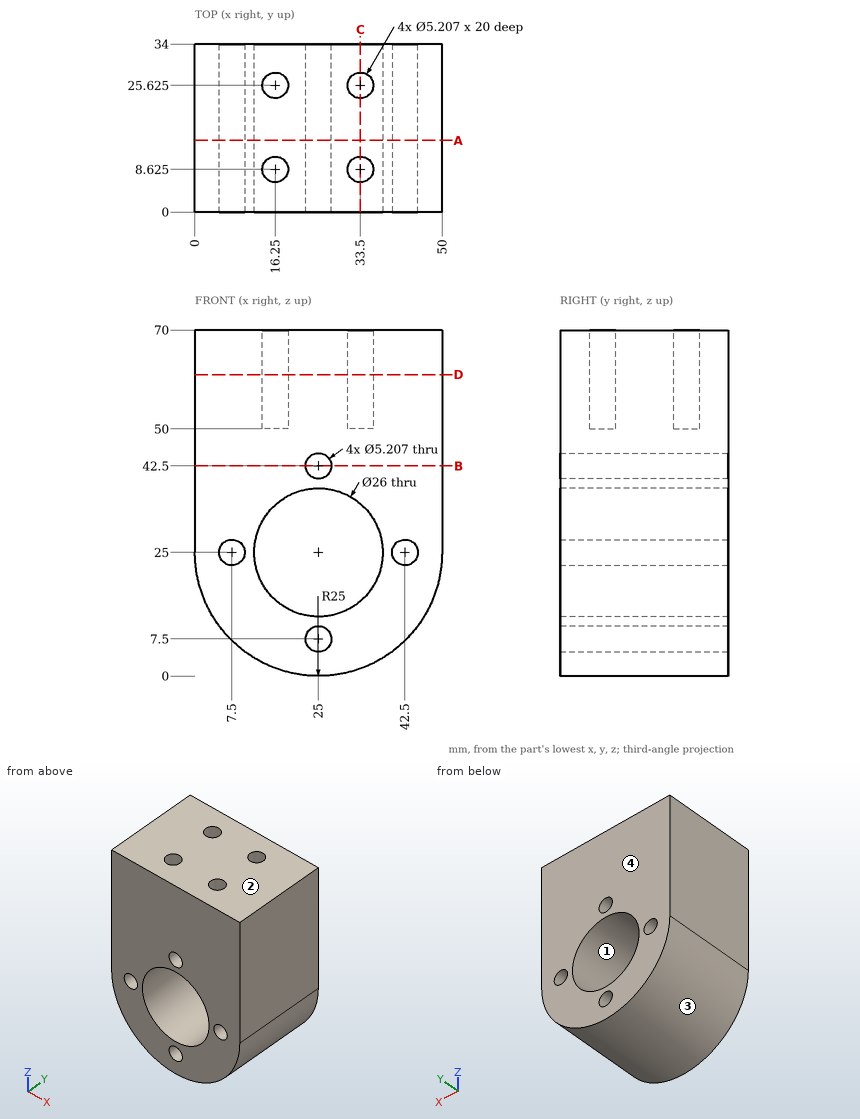
The figure shows three views and two pictorial views of one solid part (mm, origin at its lowest corner). Answer the questions. Round coordinates to 2 decimals unless told otherwise and drop trailing zeros. Loops run counter-clockwise (first coordinate to the right, second up) from the corner with the lowest first, then second, coordinate; pieces in that order, holes last. Notation, with made-up numbers: M 46.5,10.5 L 71.5,10.5 A14 ccw 71.5,35.5 Z; hole C -0.5,-26 d1. An arc over 180 degrees is marked long. Use CSV: the item, a comma, the result in double quotes.
Q1. Each of these flat-tipped pins is pushed along its axis until it touches: pin 1 (12 mm diameter, centred on x = 30.5, z = 15, fed in from +Y); pin 2 (4.5 mm diameter, centred on x = 33.5, y = 8.625, fed in from +Z); pin 3 (4 mm diameter, centred on x = 42.5, z = 25, fed in from -Y); pin 4 (4 mm diameter, centred on y = 21.5, z = 10, fed in from -X). Where does it stop, or does it pass through?
Determined:
pin 1,"y = 34"
pin 2,"z = 50"
pin 3,"through"
pin 4,"x = 3.65"
Q2. Section B-B, the plane z = 42.5 is taken. Determine the outline of the cut face in (x, y).
Determined:
outline,"M 0,0 L 22.4,0 L 22.4,34 L 0,34 Z; M 27.6,0 L 50,0 L 50,34 L 27.6,34 Z"
Q3. Section A-A, the plane y = 14.5 is taken. Determine the outline of the cut face in (x, z), then the cut area to 3 significant figures.
Determined:
outline,"M 0,25 A25 ccw 50,25 L 50,70 L 0,70 Z; hole C 7.5,25 d5.21; hole C 25,25 d26; hole C 25,7.5 d5.21; hole C 25,42.5 d5.21; hole C 42.5,25 d5.21"
area,"2,620 mm2"
Q4. Section D-D, the plane z = 61 is taken. State how many separate pieces and enclosed holes the cut face has, then the cut area to 3 significant figures.
Determined:
separate pieces,"1"
enclosed holes,"4"
area,"1,610 mm2"
Q5. Consider L1, parallel to Z at x = 24.5, y = 5 (3 decimals); L2, parallel to Y at x = 33, z = 55; L3, parallel to Z at x = 23, y = 26.5. Determine where each line is inside the solid, lowest interval first.
Determined:
L1,"0.005 to 4.945, 10.055 to 12.01, 37.99 to 39.945, 45.055 to 70"
L2,"0 to 6.07, 11.18 to 23.07, 28.18 to 34"
L3,"0.08 to 5.83, 9.17 to 12.15, 37.85 to 40.83, 44.17 to 70"
Q6. Section C-C, the plane x = 33.5 is taken. Determine the outline of the cut face in (y, z).
Determined:
outline,"M 0,1.49 L 34,1.49 L 34,15.16 L 0,15.16 Z; M 0,34.84 L 34,34.84 L 34,70 L 28.23,70 L 28.23,50 L 23.02,50 L 23.02,70 L 11.23,70 L 11.23,50 L 6.02,50 L 6.02,70 L 0,70 Z"
Q7. The mould has two halves that part along Z. Classify the marked faces 1, 2, 3 and 4: pulls with the +Z half, pulls with the -Z half, needs draft (parallel to the pull), parting line crosses it, or undercut.
Determined:
face 1,"undercut"
face 2,"pulls with the +Z half"
face 3,"pulls with the -Z half"
face 4,"needs draft"
